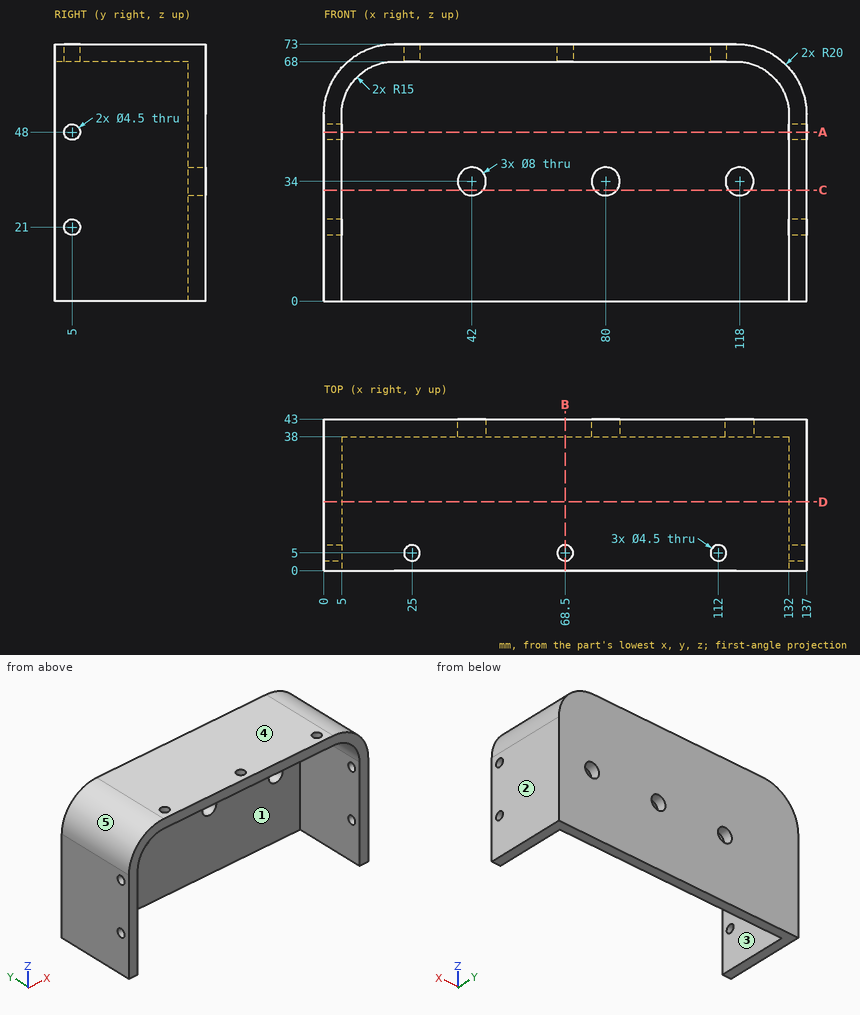
Can you work these out from the drawing? Everything is in mm from the part's minimum corner. A direction names the side the tool comes from. Give positions to 0.01 mm unless a question says otherwise; leave off trailing zeros. Order: outer loops, then holes, each group sorted by start corner. A loop starts at its lowest first (then second) coordinate and runs counter-clockwise, first axis right, second up.
1. Will these pins go through, and if not, where does the flat tip stop? P1, Ø13, axis at x = 118, z = 34, coming from the -Y side; P2, Ø10, axis at x = 74, y = 18.5, coming from the -Z side.
2. For the marked faces 1 and 2, which set-ups out of +Z, -Z, +X, -X, +Y, -Y let a thin tool reach every point of the face, with its end or its side?
3. Suppose I cut it at B-B (x = 68.5). List the corners of the cut face in (y, z) for me.
4. Suppose I cut it at C-C (z = 31.5). List the corners of the cut face in (x, y) for me.
5. Suppose I cut it at D-D (y = 19.5). List the corners of the cut face in (x, z) for me, plus the area to 3 significant figures.
6. We'd pull the mould along X, two halves only. Please class the marked faces 3, 4 and 5: pulls with the +X half, pulls with the -X half, needs draft (parallel to the pull), parting line crosses it, or undercut.
7. I need wall thicknesses on L1, parallel to X at y = 33, z = 29; L2, parallel to Z at x = 118, y = 39.45; L3, parallel to Z at x = 3.2, y = 5. Which ranges of each line are inside material? Lowest first, please.
8. Suppose I cut it at A-A (z = 48). List the corners of the cut face in (x, y) for me, plus the area to 3 significant figures.
Solved:
1. P1: stops at y = 38
1. P2: stops at z = 68
2. face 1: -Z, -Y
2. face 2: +Z, -Z, +X, +Y, -Y
3. outline: (0, 68) - (2.75, 68) - (2.75, 73) - (0, 73) - close; (7.25, 68) - (38, 68) - (38, 0) - (43, 0) - (43, 73) - (7.25, 73) - close
4. outline: (0, 0) - (5, 0) - (5, 38) - (38.88, 38) - (38.88, 43) - (0, 43) - close; (45.12, 38) - (76.88, 38) - (76.88, 43) - (45.12, 43) - close; (83.12, 38) - (114.88, 38) - (114.88, 43) - (83.12, 43) - close; (121.12, 38) - (132, 38) - (132, 0) - (137, 0) - (137, 43) - (121.12, 43) - close
5. outline: (0, 0) - (5, 0) - (5, 53) arc R15 cw to (20, 68) - (117, 68) arc R15 cw to (132, 53) - (132, 0) - (137, 0) - (137, 53) arc R20 ccw to (117, 73) - (20, 73) arc R20 ccw to (0, 53) - close
5. area: 1,290 mm2
6. face 3: undercut
6. face 4: needs draft
6. face 5: pulls with the -X half
7. L1: x = 0 to 5, 132 to 137
7. L2: z = 0 to 30, 38 to 72.97
7. L3: z = 0 to 18.75, 23.25 to 45.75, 50.25 to 63.85
8. outline: (0, 0) - (5, 0) - (5, 2.75) - (0, 2.75) - close; (0, 7.25) - (5, 7.25) - (5, 38) - (132, 38) - (132, 7.25) - (137, 7.25) - (137, 43) - (0, 43) - close; (132, 0) - (137, 0) - (137, 2.75) - (132, 2.75) - close
8. area: 1,020 mm2
